from build123d import *

# Parameters (mm, degrees)
SKETCH1_W           = 180
SKETCH1_H           = 90
BOSS_EXTRUDE1_DEPTH = 5
SKETCH2_R           = 4
CUT_EXTRUDE1_DEPTH  = 101.747208398
SKETCH3_W           = 23
SKETCH3_H           = 2.5
CUT_EXTRUDE2_DEPTH  = 101.747208398
FILLET1_R           = 3
FILLET2_R           = 3
FILLET3_R           = 3
FILLET4_R           = 3
SKETCH4_W           = 13.5
SKETCH4_H           = 21
CUT_EXTRUDE3_DEPTH  = 101.747208398


with BuildPart() as part:
    # Sketch1 → Boss-Extrude1 (new body)
    with BuildSketch(Plane.XY):
        Rectangle(SKETCH1_W, SKETCH1_H)
    extrude(amount=BOSS_EXTRUDE1_DEPTH)

    # Sketch2 → Cut-Extrude1 (cut, through all)
    with BuildSketch(Plane.XY.offset(5)):
        with Locations((-81, 36)):
            Circle(SKETCH2_R)
        with Locations(Location((81, 36, 0), (0, 0, 180))):
            Circle(SKETCH2_R)
        with Locations((81, -36)):
            Circle(SKETCH2_R)
        with Locations(Location((-81, -36, 0), (0, 0, 180))):
            Circle(SKETCH2_R)
    extrude(amount=-CUT_EXTRUDE1_DEPTH, mode=Mode.SUBTRACT)

    # Sketch3 → Cut-Extrude2 (cut, through all)
    with BuildSketch(Plane(origin=(0, 0, 0), x_dir=(-1, 0, 0), z_dir=(0, 0, -1))):
        Rectangle(SKETCH3_W, SKETCH3_H)
    extrude(amount=-CUT_EXTRUDE2_DEPTH, mode=Mode.SUBTRACT)

    # Fillet1
    fillet1_edges = [part.edges().sort_by_distance(p)[0] for p in [
        (90, 45, 2.5),
    ]]
    fillet(fillet1_edges, radius=FILLET1_R)

    # Fillet2
    fillet2_edges = [part.edges().sort_by_distance(p)[0] for p in [
        (90, -45, 2.5),
    ]]
    fillet(fillet2_edges, radius=FILLET2_R)

    # Fillet3
    fillet3_edges = [part.edges().sort_by_distance(p)[0] for p in [
        (-90, 45, 2.5),
    ]]
    fillet(fillet3_edges, radius=FILLET3_R)

    # Fillet4
    fillet4_edges = [part.edges().sort_by_distance(p)[0] for p in [
        (-90, -45, 2.5),
    ]]
    fillet(fillet4_edges, radius=FILLET4_R)

    # Sketch4 → Cut-Extrude3 (cut, through all)
    with BuildSketch(Plane.XY.offset(5)):
        with Locations((45, 0)):
            Rectangle(SKETCH4_W, SKETCH4_H)
    extrude(amount=-CUT_EXTRUDE3_DEPTH, mode=Mode.SUBTRACT)


solid = part.part
Input: part model. Units: mm. Frame: model coordinates. A direction names the side the tool comes from. Coordinates: 2 decimals unless noted, no trailing zeros. Loops run counter-clockwise (first coordinate to the right, second up) from the corner with the lowest first, then second, coordinate; pieces in that order, holes last.
(1) Section B-B on x = -81. Return the cut outline in (y, z).
(2) Section C-C on z = 1.5. Return the cut outline in (x, y), then the cut area to 3 significant figures.
(3) Material intervals for probe 1 along Y at (x, z) = (81, 3.55); probe 2 along X at (y, z) = (36.5, 3.3); probe 3 along Y at (x, z) = (-3, 2.2), sorted ascending.
(4) Section A-A on y = 36. Return the cut outline in (x, z), then the cut area to 3 significant figures.
(5) Section D-D on x = 49.5. Return the cut outline in (y, z), then the cut area to 3 significant figures.
(6) Pull-direction query (X, two-part tool) for faces 3 (the face through (90, -1, 2)), 4 (the face through (51.75, 0, 3)), 5 (the face through (-81.521, 39.966, 2.535)), 6 (the face through (-1, 11, 0)); classes: released by +X, released by -X, zero draft, split by the parting line, or undercut.
(7) Set-up query: faces 1 (the face through (45, -10.5, 3)), 2 (the face through (-90, -1, 2)). Return all of +Z, -Z, +X, -X, +Y, -Y with unobstructed straight access to the full face (end or side cutting, diameter ignored); none if empty.
Data:
1. outline: (-45, 0) - (-40, 0) - (-40, 5) - (-45, 5) - close; (-32, 0) - (32, 0) - (32, 5) - (-32, 5) - close; (40, 0) - (45, 0) - (45, 5) - (40, 5) - close
2. outline: (-90, -42) arc R3 ccw to (-87, -45) - (87, -45) arc R3 ccw to (90, -42) - (90, 42) arc R3 ccw to (87, 45) - (-87, 45) arc R3 ccw to (-90, 42) - close; hole circle Ø8 at (-81, -36); hole circle Ø8 at (-81, 36); hole (-11.5, -1.25) - (11.5, -1.25) - (11.5, 1.25) - (-11.5, 1.25) - close; hole (38.25, -10.5) - (51.75, -10.5) - (51.75, 10.5) - (38.25, 10.5) - close; hole circle Ø8 at (81, -36); hole circle Ø8 at (81, 36)
2. area: 15,700 mm2
3. probe 1: y = -45 to -40, -32 to 32, 40 to 45
3. probe 2: x = -90 to -84.97, -77.03 to 77.03, 84.97 to 90
3. probe 3: y = -45 to -1.25, 1.25 to 45
4. outline: (-90, 0) - (-85, 0) - (-85, 5) - (-90, 5) - close; (-77, 0) - (77, 0) - (77, 5) - (-77, 5) - close; (85, 0) - (90, 0) - (90, 5) - (85, 5) - close
4. area: 820 mm2
5. outline: (-45, 0) - (-10.5, 0) - (-10.5, 5) - (-45, 5) - close; (10.5, 0) - (45, 0) - (45, 5) - (10.5, 5) - close
5. area: 345 mm2
6. face 3: released by +X
6. face 4: undercut
6. face 5: undercut
6. face 6: zero draft
7. face 1: +Z, -Z
7. face 2: +Z, -Z, -X, +Y, -Y
